Design review of the part built by this model. Coordinates are the model's own, in mm. Give positions to 0.01 mm unless a question says otherwise; leave off trailing zeros. Loops run counter-clockwise (first coordinate to the right, second up) from the corner with the lowest first, then second, coordinate; pieces in that order, holes last. Notation, with made-up numbers: M -7.75,26.5 L 41.25,26.5 A13 cw 41.25,36.5 Z; hole C -18,6.5 d3. An arc over 180 degrees is marked long. Use one line per item in the form item = value. Start each with the question number.
from build123d import *

# Parameters (mm, degrees)
OUTER_CASING_DEPTH = 5
SKETCH1_R          = 14.3
INNER_CUTOUT_DEPTH = 10


with BuildPart() as part:
    # Plate shape → Outer casing (new body)
    with BuildSketch(Plane.XY):
        with BuildLine():
            Line((-175, 225), (-175, 0))
            Line((-175, 0), (175, 0))
            Line((175, 0), (175, 225))
            ThreePointArc((175, 225), (0, 400), (-175, 225))
        make_face()
    extrude(amount=OUTER_CASING_DEPTH)

    # Sketch1 → Inner Cutout (cut)
    with BuildSketch(Plane.XY.offset(5)):
        with Locations((0, 225)):
            Circle(SKETCH1_R)
    extrude(amount=-INNER_CUTOUT_DEPTH, mode=Mode.SUBTRACT)


solid = part.part
Q1. The part is to be moulded in two halves that separate along X. For faces 1 (the cylindrical face through (-1.86, 239.18, 2.54)), 2 (the cylindrical face through (3.848, 399.958, 2.465)), 3 (the flat face through (-2, 203, 0)), say which applies: pulls with the +X half, pulls with the -X half, needs draft (parallel to the pull), parting line crosses it, or undercut.
Q2. Wall thickness on probe 1 along Y at (x, z) = (0, 2.7); probe 2 along Y at (x, z) = (10, 3); probe 3 along Y at (x, z) = (142.5, 4.35): over which ranges is each line inside the solid? List them lowest first.
Q3. Take a section at D-D on x = -149.5. Give the boundary of the cut face in (y, z), plus the area to 3 significant figures.
Q4. Clearance check with flat-ended pins moving along their axes: pin 1 Ø2 at (y, z) = (256, 1) entering from -X; pin 2 Ø3 at (x, y) = (-70, 250) entering from -Z. State where each tip first meets the part, or that it passes through.
Q5. Take a section at C-C on y = 301. Give the boundary of the cut face in (x, z).
Q6. Take a section at B-B on z = 3.45. Give the boundary of the cut face in (x, y).
Q7. Take a section at A-A on x = 0. Give the boundary of the cut face in (y, z).
Response values:
q1.face_1 = undercut
q1.face_2 = parting line crosses it
q1.face_3 = needs draft
q2.probe_1 = 0 to 210.7, 239.3 to 400
q2.probe_2 = 0 to 214.78, 235.22 to 399.71
q2.probe_3 = 0 to 326.58
q3.outline = M 0,0 L 315.97,0 L 315.97,5 L 0,5 Z
q3.area = 1,580 mm^2
q4.pin_1 = -172.41
q4.pin_2 = 0
q5.outline = M -157.64,0 L 157.64,0 L 157.64,5 L -157.64,5 Z
q6.outline = M -175,0 L 175,0 L 175,225 A175 ccw -175,225 Z; hole C 0,225 d28.6
q7.outline = M 0,0 L 210.7,0 L 210.7,5 L 0,5 Z; M 239.3,0 L 400,0 L 400,5 L 239.3,5 Z
